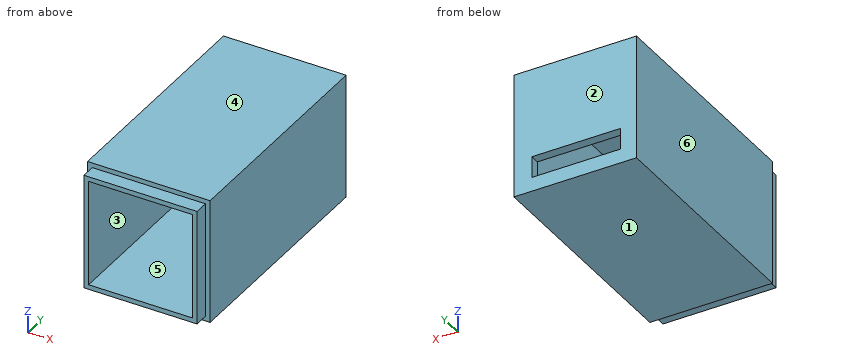
```python
from build123d import *

# Parameters (mm, degrees)
EXTRUDE_1_DEPTH      = 17
EXTRUDE_1_DEPTH_BACK = 5.5
SKETCH_2_W           = 26
SKETCH_2_H           = 51
SKETCH_2_W_2         = 22
SKETCH_2_H_2         = 47
SKETCH_3_W           = 26
SKETCH_3_H           = 51
EXTRUDE_2_DEPTH      = 2
CUT_EXTRUDE_START    = -17
SKETCH_4_W           = 18.8
SKETCH_4_H           = 2
CUT_EXTRUDE_1_DEPTH  = 4.5
SKETCH_5_W           = 26
SKETCH_5_H           = 51
EXTRUDE_3_DEPTH      = 2
SKETCH_6_W           = 26
SKETCH_6_H           = 26.5
CUT_EXTRUDE_2_DEPTH  = 2
SKETCH_7_W           = 24
SKETCH_7_H           = 24.5
SKETCH_7_W_2         = 22
SKETCH_7_H_2         = 22.5
EXTRUDE_4_DEPTH      = 3


with BuildPart() as part:
    # 草图2 → 凸台-拉伸1 (new, two sides: drawn at the far end of the back side and taken through both)
    with BuildSketch(Plane.XY.offset(-EXTRUDE_1_DEPTH_BACK)):
        with Locations((11, 23.5)):
            Rectangle(SKETCH_2_W, SKETCH_2_H)
        with Locations((11, 23.5)):
            Rectangle(SKETCH_2_W_2, SKETCH_2_H_2, mode=Mode.SUBTRACT)
    extrude(amount=EXTRUDE_1_DEPTH + EXTRUDE_1_DEPTH_BACK)

    # 草图3 → 凸台-拉伸2 (add)
    with BuildSketch(Plane(origin=(0, 0, -5.5), x_dir=(-1, 0, 0), z_dir=(0, 0, -1))):
        with Locations((-11, 23.5)):
            Rectangle(SKETCH_3_W, SKETCH_3_H)
    extrude(amount=EXTRUDE_2_DEPTH)

    # 草图4 → 切除-拉伸1 (cut)
    with BuildSketch(Plane.XY.offset(17).offset(CUT_EXTRUDE_START)):
        with Locations((10.8, 48)):
            Rectangle(SKETCH_4_W, SKETCH_4_H)
    extrude(amount=-CUT_EXTRUDE_1_DEPTH, mode=Mode.SUBTRACT)

    # 草图5 → 凸台-拉伸3 (add)
    with BuildSketch(Plane.XY.offset(17)):
        with Locations((11, 23.5)):
            Rectangle(SKETCH_5_W, SKETCH_5_H)
    extrude(amount=EXTRUDE_3_DEPTH)

    # 草图6 → 切除-拉伸2 (cut)
    with BuildSketch(Plane.XZ.offset(2)):
        with Locations((11, 5.75)):
            Rectangle(SKETCH_6_W, SKETCH_6_H)
    extrude(amount=-CUT_EXTRUDE_2_DEPTH, mode=Mode.SUBTRACT)

    # 草图7 → 凸台-拉伸4 (add)
    with BuildSketch(Plane.XZ):
        with Locations((11, 5.750930711)):
            Rectangle(SKETCH_7_W, SKETCH_7_H)
        with Locations((11, 5.75)):
            Rectangle(SKETCH_7_W_2, SKETCH_7_H_2, mode=Mode.SUBTRACT)
    extrude(amount=EXTRUDE_4_DEPTH)


solid = part.part
```
Geometry: final body of the model. Coordinates: model frame, mm. Face numbers are marked on the shaded views. A direction names the side the tool comes from. Coordinates: 2 decimals unless noted, no trailing zeros. Order: outer loops, then holes, each group sorted by start corner. A loop starts at its lowest first (then second) coordinate and runs counter-clockwise, first axis right, second up. Notation, with made-up numbers: (83.25, 20.25) -> (131.25, 20.25) arc R22 ccw to (131.25, 53.25) -> close; hole circle Ø9 at (85, 47). An arc over 180 degrees is marked (long way). Answer in a Markdown table with one row per item.
Item 1: Draft query along Z for the marked faces 1, 2, 3 and 4. Return one class per face: released by +Z, released by -Z, zero draft, split by the parting line, or undercut.
Return value:
| item | result |
|---|---|
| face 1 | released by -Z |
| face 2 | zero draft |
| face 3 | undercut |
| face 4 | released by +Z |
Item 2: Contact query for flat-ended pins moving along their axis: P1, Ø1.5, axis at y = -1, z = 11, coming from the +X side; P2, Ø0.9, axis at x = 11.5, y = -1.5, coming from the +Z side; P3, Ø2.5, axis at y = -2, z = 0, coming from the -X side. Output: stop coordinate, or through.
Return value:
| item | result |
|---|---|
| P1 | stops at x = 23 |
| P2 | stops at z = 18 |
| P3 | stops at x = -1 |
Item 3: Section A-A on y = 15.5. Output: boundary loops of the cut face in (x, z).
Return value:
| item | result |
|---|---|
| outline | (-2, -7.5) -> (24, -7.5) -> (24, 19) -> (-2, 19) -> close; hole (0, -5.5) -> (22, -5.5) -> (22, 17) -> (0, 17) -> close |
Item 4: Ray query, L1, parallel to X at y = 12.5, z = 3.25; L2, parallel to Z at x = 14.25, y = 12.5; L3, parallel to X at y = -1, z = 14.75. Return the intervals inside material, ascending.
Return value:
| item | result |
|---|---|
| L1 | x = -2 to 0, 22 to 24 |
| L2 | z = -7.5 to -5.5, 17 to 19 |
| L3 | x = -1 to 0, 22 to 23 |
Item 5: Access query for the marked faces 5 and 6. Directions: +Z, -Z, +X, -X, +Y, -Y. A direction counts if a zero-diameter tool reaches every point of the face in a straight line with its end or side. Return the directions, or none.
Return value:
| item | result |
|---|---|
| face 5 | -Y |
| face 6 | +Z, -Z, -X, +Y, -Y |
Item 6: Section C-C on z = 3.5. Output: boundary loops of the cut face in (x, y).
Return value:
| item | result |
|---|---|
| outline | (-2, 0) -> (-1, 0) -> (-1, -3) -> (0, -3) -> (0, 47) -> (22, 47) -> (22, -3) -> (23, -3) -> (23, 0) -> (24, 0) -> (24, 49) -> (-2, 49) -> close |
Item 7: Section D-D on x = 21. Output: boundary loops of the cut face in (y, z), plus the area to 3 significant figures.
Return value:
| item | result |
|---|---|
| outline | (-3, -6.5) -> (0, -6.5) -> (0, -7.5) -> (49, -7.5) -> (49, 19) -> (0, 19) -> (0, 18) -> (-3, 18) -> (-3, 17) -> (47, 17) -> (47, -5.5) -> (-3, -5.5) -> close |
| area | 247 mm² |
Item 8: Section B-B on x = 7.5. Output: boundary loops of the cut face in (y, z), plus the area to 3 significant figures.
Return value:
| item | result |
|---|---|
| outline | (-3, -6.5) -> (0, -6.5) -> (0, -7.5) -> (49, -7.5) -> (49, -4.5) -> (47, -4.5) -> (47, -5.5) -> (-3, -5.5) -> close; (-3, 17) -> (47, 17) -> (47, 0) -> (49, 0) -> (49, 19) -> (0, 19) -> (0, 18) -> (-3, 18) -> close |
| area | 238 mm² |
